from build123d import *

# Parameters (mm, degrees)
SKETCH_W        = 100
SKETCH_H        = 84
PAD_DEPTH       = 10
SKETCH001_R     = 2.1
POCKET_DEPTH    = 10
SKETCH002_R     = 3.2
POCKET001_DEPTH = 10
SKETCH003_R     = 4
POCKET002_DEPTH = 5
POCKET003_DEPTH = 4
POCKET004_DEPTH = 5.2


with BuildPart() as part:
    # Sketch → Pad (new body)
    with BuildSketch(Plane.XY):
        with Locations((50, 42)):
            Rectangle(SKETCH_W, SKETCH_H)
    extrude(amount=PAD_DEPTH)

    # Sketch001 (on Face6 of Pad) → Pocket (cut)
    with BuildSketch(Plane.XY.offset(10)):
        with Locations((6, 78)):
            Circle(SKETCH001_R)
        with Locations((30, 78)):
            Circle(SKETCH001_R)
        with Locations((6, 60)):
            Circle(SKETCH001_R)
        with Locations((30, 60)):
            Circle(SKETCH001_R)
        with Locations((6, 24)):
            Circle(SKETCH001_R)
        with Locations((30, 24)):
            Circle(SKETCH001_R)
        with Locations((6, 6)):
            Circle(SKETCH001_R)
        with Locations((30, 6)):
            Circle(SKETCH001_R)
        with Locations((70, 78)):
            Circle(SKETCH001_R)
        with Locations((94, 78)):
            Circle(SKETCH001_R)
        with Locations((70, 60)):
            Circle(SKETCH001_R)
        with Locations((94, 60)):
            Circle(SKETCH001_R)
        with Locations((70, 24)):
            Circle(SKETCH001_R)
        with Locations((94, 24)):
            Circle(SKETCH001_R)
        with Locations((70, 6)):
            Circle(SKETCH001_R)
        with Locations((94, 6)):
            Circle(SKETCH001_R)
        with Locations((35, 47)):
            Circle(SKETCH001_R)
        with Locations((65, 47)):
            Circle(SKETCH001_R)
        with Locations((35, 37)):
            Circle(SKETCH001_R)
        with Locations((65, 37)):
            Circle(SKETCH001_R)
    extrude(amount=-POCKET_DEPTH, mode=Mode.SUBTRACT)

    # Sketch002 (on Face5 of Pocket) → Pocket001 (cut)
    with BuildSketch(Plane.XY.offset(10)):
        with Locations((20, 62)):
            Circle(SKETCH002_R)
        with Locations((20, 22)):
            Circle(SKETCH002_R)
        with Locations((80, 62)):
            Circle(SKETCH002_R)
        with Locations((80, 22)):
            Circle(SKETCH002_R)
    extrude(amount=-POCKET001_DEPTH, mode=Mode.SUBTRACT)

    # Sketch003 (on Face5 of Pocket001) → Pocket002 (cut)
    with BuildSketch(Plane.XY.offset(10)):
        with Locations((6, 78)):
            Circle(SKETCH003_R)
        with Locations((30, 78)):
            Circle(SKETCH003_R)
        with Locations((30, 60)):
            Circle(SKETCH003_R)
        with Locations((6, 60)):
            Circle(SKETCH003_R)
        with Locations((70, 78)):
            Circle(SKETCH003_R)
        with Locations((94, 78)):
            Circle(SKETCH003_R)
        with Locations((70, 60)):
            Circle(SKETCH003_R)
        with Locations((94, 60)):
            Circle(SKETCH003_R)
        with Locations((6, 24)):
            Circle(SKETCH003_R)
        with Locations((30, 24)):
            Circle(SKETCH003_R)
        with Locations((6, 6)):
            Circle(SKETCH003_R)
        with Locations((30, 6)):
            Circle(SKETCH003_R)
        with Locations((70, 24)):
            Circle(SKETCH003_R)
        with Locations((94, 24)):
            Circle(SKETCH003_R)
        with Locations((70, 6)):
            Circle(SKETCH003_R)
        with Locations((94, 6)):
            Circle(SKETCH003_R)
        with Locations((35, 47)):
            Circle(SKETCH003_R)
        with Locations((35, 37)):
            Circle(SKETCH003_R)
        with Locations((65, 37)):
            Circle(SKETCH003_R)
        with Locations((65, 47)):
            Circle(SKETCH003_R)
    extrude(amount=-POCKET002_DEPTH, mode=Mode.SUBTRACT)

    # Sketch003 (on Face5 of Pocket001) → Pocket003 (cut)
    with BuildSketch(Plane.XY.offset(10)):
        with Locations((6, 78)):
            Circle(SKETCH003_R)
        with Locations((30, 78)):
            Circle(SKETCH003_R)
        with Locations((30, 60)):
            Circle(SKETCH003_R)
        with Locations((6, 60)):
            Circle(SKETCH003_R)
        with Locations((70, 78)):
            Circle(SKETCH003_R)
        with Locations((94, 78)):
            Circle(SKETCH003_R)
        with Locations((70, 60)):
            Circle(SKETCH003_R)
        with Locations((94, 60)):
            Circle(SKETCH003_R)
        with Locations((6, 24)):
            Circle(SKETCH003_R)
        with Locations((30, 24)):
            Circle(SKETCH003_R)
        with Locations((6, 6)):
            Circle(SKETCH003_R)
        with Locations((30, 6)):
            Circle(SKETCH003_R)
        with Locations((70, 24)):
            Circle(SKETCH003_R)
        with Locations((94, 24)):
            Circle(SKETCH003_R)
        with Locations((70, 6)):
            Circle(SKETCH003_R)
        with Locations((94, 6)):
            Circle(SKETCH003_R)
        with Locations((35, 47)):
            Circle(SKETCH003_R)
        with Locations((35, 37)):
            Circle(SKETCH003_R)
        with Locations((65, 37)):
            Circle(SKETCH003_R)
        with Locations((65, 47)):
            Circle(SKETCH003_R)
    extrude(amount=-POCKET003_DEPTH, mode=Mode.SUBTRACT)

    # Sketch004 (on Face4 of Pocket003) → Pocket004 (cut)
    with BuildSketch(Plane(origin=(0, 0, 0), x_dir=(1, 0, 0), z_dir=(0, 0, -1))):
        Polygon((14.42356, -23.704889), (18.688257, -27.681783), (24.264697, -25.976895), (25.57644, -20.295111), (21.311743, -16.318217), (15.735303, -18.023105), align=None)
        Polygon((74.318217, -20.688257), (76.023105, -26.264697), (81.704889, -27.57644), (85.681783, -23.311743), (83.976895, -17.735303), (78.295111, -16.42356), align=None)
        Polygon((74.42356, -63.704889), (78.688257, -67.681783), (84.264697, -65.976895), (85.57644, -60.295111), (81.311743, -56.318217), (75.735303, -58.023105), align=None)
        Polygon((14.318217, -60.688257), (16.023105, -66.264697), (21.704889, -67.57644), (25.681783, -63.311743), (23.976895, -57.735303), (18.295111, -56.42356), align=None)
    extrude(amount=-POCKET004_DEPTH, mode=Mode.SUBTRACT)


solid = part.part
Design review of the part built by this model. Coordinates are the model's own, in mm. A direction names the side the tool comes from. Give positions to 0.01 mm unless a question says otherwise; leave off trailing zeros. Answer as a JSON object with one key per item and string values. Group by question number.
1) We need section A-A (z = 7.75). Count the separate pieces of the cut face and the enclosed holes in it, and give its area (3 significant figures).
2) For line 1 along Y through (x, z) = (80, 8.7); line 2 along Y through (x, z) = (70, 8.35); line 3 along Y through (x, z) = (19.5, 4.5), list the stretches that pass through material, from the lowest coordinate up.
3) Tool access review of faces 3 (the face through (24.91, 23.18, 2.56)), 4 (the face through (68.695, 45.468, 7.535)), 5 (the face through (71.13, 25.77, 2.54)): name each direction out of +Z, -Z, +X, -X, +Y, -Y from which nothing blocks a thin tool from reaching the whole face with its end or side.
4) Clearance check with flat-ended pins moving along their axes: pin 1 Ø10 at (x, y) = (20, 22) entering from -Z; pin 2 Ø2.5 at (x, y) = (69, 62) entering from +Z. State where each tip first meets the part, or that it passes through.
5) Mouldability with a two-part tool opening along X and no side actions: class faces 1 (the face through (96, 4, 5)), 2 (the face through (23.67, 65.47, 2.56)) as released by +X, released by -X, zero draft, split by the parting line, or undercut.
Answer key:
{
 "1": {"separate pieces": "1", "enclosed holes": "24", "area": "7,270 mm²"},
 "2": {"line 1": "y = 0 to 18.8, 25.2 to 58.8, 65.2 to 84", "line 2": "y = 0 to 2, 10 to 20, 28 to 56, 64 to 74, 82 to 84", "line 3": "y = 0 to 16.87, 27.43 to 56.7, 67.07 to 84"},
 "3": {"face 3": "-Z", "face 4": "+Z", "face 5": "+Z, -Z"},
 "4": {"pin 1": "stops at z = 5.2", "pin 2": "stops at z = 5"},
 "5": {"face 1": "undercut", "face 2": "undercut"}
}
